from build123d import *

# Parameters (mm, degrees)
CROQUIS2_W              = 45
CROQUIS2_H              = 15
SALIENTE_EXTRUIR1_DEPTH = 5
REDONDEO1_R             = 3
CROQUIS3_R              = 4
CORTAR_EXTRUIR1_DEPTH   = 10


with BuildPart() as part:
    # Croquis2 → Saliente-Extruir1 (new body)
    with BuildSketch(Plane(origin=(0, 0, 0), x_dir=(1, 0, 0), z_dir=(0, 1, 0))):
        Rectangle(CROQUIS2_W, CROQUIS2_H)
    extrude(amount=SALIENTE_EXTRUIR1_DEPTH)

    # Redondeo1
    redondeo1_edges = [part.edges().sort_by_distance(p)[0] for p in [
        (22.5, 2.5, 7.5),
        (-22.5, 2.5, 7.5),
        (-22.5, 2.5, -7.5),
        (22.5, 2.5, -7.5),
    ]]
    fillet(redondeo1_edges, radius=REDONDEO1_R)

    # Croquis3 → Cortar-Extruir1 (cut, symmetric)
    with BuildSketch(Plane(origin=(0, 5, 0), x_dir=(1, 0, 0), z_dir=(0, 1, 0))):
        with Locations(Location((-15, 0, 0), (0, 0, 90))):
            Circle(CROQUIS3_R)
        with Locations(Location((15, 0, 0), (0, 0, 90))):
            Circle(CROQUIS3_R)
    extrude(amount=CORTAR_EXTRUIR1_DEPTH, both=True, mode=Mode.SUBTRACT)


solid = part.part
Verification items for the finished model (mm, model axes). Coordinates: 2 decimals unless noted, no trailing zeros. Order: outer loops, then holes, each group sorted by start corner. A loop starts at its lowest first (then second) coordinate and runs counter-clockwise, first axis right, second up.
Item 1: Section check A-A, the plane z = 0. Enter the section's corners in (x, y), then the cut area to 3 significant figures.
Filled in:
outline: (-22.5, 0) - (-19, 0) - (-19, 5) - (-22.5, 5) - close; (-11, 0) - (11, 0) - (11, 5) - (-11, 5) - close; (19, 0) - (22.5, 0) - (22.5, 5) - (19, 5) - close
area: 145 mm2
Item 2: Section check B-B, the plane x = -15. Enter the section's corners in (y, z), then the cut area to 3 significant figures.
Filled in:
outline: (0, -7.5) - (5, -7.5) - (5, -4) - (0, -4) - close; (0, 4) - (5, 4) - (5, 7.5) - (0, 7.5) - close
area: 35.0 mm2
Item 3: Section check D-D, the plane z = 2.5. Enter the section's corners in (x, y).
Filled in:
outline: (-22.5, 0) - (-18.12, 0) - (-18.12, 5) - (-22.5, 5) - close; (-11.88, 0) - (11.88, 0) - (11.88, 5) - (-11.88, 5) - close; (18.12, 0) - (22.5, 0) - (22.5, 5) - (18.12, 5) - close
Item 4: Material ranges on L1, parallel to X at y = 3.75, z = 0; L2, parallel to Z at x = -15, y = 4; L3, parallel to X at y = 2.4, z = 2.5, recorded low to high.
Filled in:
L1: x = -22.5 to -19, -11 to 11, 19 to 22.5
L2: z = -7.5 to -4, 4 to 7.5
L3: x = -22.5 to -18.12, -11.88 to 11.88, 18.12 to 22.5
Item 5: Release check for a two-part mould opening along X. For faces 1 (the face through (11.034, 2.535, 0.521)), 2 (the face through (0, 2, 7.5)), 3 (the face through (-21.64, 2.54, 6.6)), 4 (the face through (-18.966, 2.535, 0.521)) record: +X half, -X half, draft (parallel to the pull), parting line (faces both ways), or undercut.
Filled in:
face 1: undercut
face 2: draft
face 3: -X half
face 4: undercut
Item 6: Section check C-C, the plane y = 1.95. Enter the section's corners in (x, z), then the cut area to 3 significant figures.
Filled in:
outline: (-22.5, -4.5) arc R3 ccw to (-19.5, -7.5) - (19.5, -7.5) arc R3 ccw to (22.5, -4.5) - (22.5, 4.5) arc R3 ccw to (19.5, 7.5) - (-19.5, 7.5) arc R3 ccw to (-22.5, 4.5) - close; hole circle Ø8 at (-15, 0); hole circle Ø8 at (15, 0)
area: 567 mm2
